Model file for the job. Use its own axes, mm. A direction names the side the tool comes from. Give positions to 0.01 mm unless a question says otherwise; leave off trailing zeros. Order: outer loops, then holes, each group sorted by start corner. A loop starts at its lowest first (then second) coordinate and runs counter-clockwise, first axis right, second up. Notation, with made-up numbers: (83, 45) -> (122, 45) arc R31 cw to (122, 83) -> close; hole circle Ø4 at (61, 49.5). An arc over 180 degrees is marked (long way). Use CSV: the item, a comma, the result in double quotes. Start each with the question number.
1. Cut at D-D on z = -6.75. List the corners of the cut face in (x, y).
2. Drop flat-ended pins along their axis: pin 1 (2.5 mm diameter, centred on x = 0, y = -67, fed in from +Z); pin 2 (4 mm diameter, centred on x = -6, y = -42.5, fed in from -Z); pin 3 (10 mm diameter, centred on y = -24, z = -1.5, fed in from -X); pin 4 (4 mm diameter, centred on x = 2, y = -69.5, fed in from -Z). Give the stop position or say it passes through.
3. Wall check: line 1 (X direction, y = -40.5, z = 10); line 2 (Y direction, x = 0.75, z = -2); line 3 (Y direction, x = -6.25, z = -7.75). Give the ranges that are in metal, low to high. Write a range as from..to.
4. 3-axis set-ups, long thin cutter, end or side, ignore diameter. For faces 4 (the flat face through (0, -75, -5)), 5 (the cylindrical face through (-7.493, -62.325, 0.33)): which of +Z, -Z, +X, -X, +Y, -Y reach the whole face in a straight line?
5. Cut at B-B on x = 0. List the corners of the cut face in (y, z), then the cut area to 4 significant figures.
6. Cut at C-C on y = -13. List the corners of the cut face in (x, z), then the cut area to 3 significant figures.
7. Pull direction X, two halves, no side cores. Call faces 1 (the flat face through (4, -68, 0)), 2 (the flat face through (3, -10, -3)), 3 (the cylindrical face through (-3, -5, 0)): released by +X, released by -X, zero draft, split by the parting line, or undercut.
8. Cut at A-A on z = 0. List the corners of the cut face in (x, y), then the cut area to 4 significant figures.
```python
from build123d import *

# Parameters (mm, degrees)
F0_R     = 3
F1_DEPTH = 10
F2_R     = 12.5
F2_R_2   = 3
F3_DEPTH = 40
F4_R     = 7.5
F5_DEPTH = 25
F6_W     = 8
F6_H     = 8
F7_DEPTH = 15


with BuildPart() as f1:
    # F0 (on Front) → F1 (new body)
    with BuildSketch(Plane.XZ):
        Circle(F0_R)
    extrude(amount=F1_DEPTH)

    # F2 (on face) → F3 (join)
    with BuildSketch(Plane.XZ.offset(10)):
        Circle(F2_R)
        Circle(F2_R_2, mode=Mode.SUBTRACT)
        Circle(F2_R_2)
    extrude(amount=F3_DEPTH)

    # F4 (on face) → F5 (join)
    with BuildSketch(Plane.XZ.offset(50)):
        Circle(F4_R)
    extrude(amount=F5_DEPTH)

    # F6 (on face) → F7 (cut)
    with BuildSketch(Plane.XZ.offset(75)):
        Rectangle(F6_W, F6_H)
    extrude(amount=-F7_DEPTH, mode=Mode.SUBTRACT)


solid = f1.part
```
Verdict:
1,outline,"(-10.52, -50) -> (-3.27, -50) -> (-3.27, -75) -> (3.27, -75) -> (3.27, -50) -> (10.52, -50) -> (10.52, -10) -> (-10.52, -10) -> close"
2,pin 1,"z = 7.5"
2,pin 2,"z = -11.84"
2,pin 3,"x = -12.5"
2,pin 4,"z = -7.5"
3,line 1,"-7.5..7.5"
3,line 2,"-60..0"
3,line 3,"-50..-10"
4,face 4,"+Z, -Z, +X, -X, -Y"
4,face 5,"-Y"
5,outline,"(-75, -7.5) -> (-50, -7.5) -> (-50, -12.5) -> (-10, -12.5) -> (-10, -3) -> (0, -3) -> (0, 3) -> (-10, 3) -> (-10, 12.5) -> (-50, 12.5) -> (-50, 7.5) -> (-75, 7.5) -> (-75, 4) -> (-60, 4) -> (-60, -4) -> (-75, -4) -> close"
5,area,"1,315 mm^2"
6,outline,"circle Ø25 at (0, 0)"
6,area,"491 mm^2"
7,face 1,"undercut"
7,face 2,"zero draft"
7,face 3,"split by the parting line"
8,outline,"(-12.5, -50) -> (-7.5, -50) -> (-7.5, -75) -> (-4, -75) -> (-4, -60) -> (4, -60) -> (4, -75) -> (7.5, -75) -> (7.5, -50) -> (12.5, -50) -> (12.5, -10) -> (3, -10) -> (3, 0) -> (-3, 0) -> (-3, -10) -> (-12.5, -10) -> close"
8,area,"1,315 mm^2"
